Geometry check sheet. Reference: the model listing, model coordinates, mm. A direction names the side the tool comes from. Coordinates: 2 decimals unless noted, no trailing zeros. Write each loop counter-clockwise with the first axis right and the second up, starting at its lowest first coordinate (ties: lowest second). Pieces come first, ordered by that corner, then holes.
Autodesk Inventor part; units mm, degrees
ref_plane "Start Plane" through (0, 0, 0) normal (0, 0, 1) x (1, 0, 0)
ref_plane "End Plane" through (0, 0, 494.9747) normal (0, 0, 1) x (1, 0, 0)
ref_plane "Work Plane4" through (12.7, 0, 494.9747) normal (0, 0.3827, 0.9239) x (1, 0, 0)
ref_plane "Start Plane" through (0, 0, 0) normal (0, 0, 1) x (1, 0, 0)
ref_plane "End Plane" through (0, 0, 494.9747) normal (0, 0, 1) x (1, 0, 0)
sketch "Sketch" plane through (0, 0, 0) normal (0, 0, 1) x (1, 0, 0)
  line L0 (25.4, 0) -> (0, 0)
  line L1 (0, 0) -> (0, 25.4)
  line L2 (0, 25.4) -> (1.651, 25.4)
  line L3 (3.175, 23.876) -> (3.175, 6.477)
  line L4 (6.477, 3.175) -> (23.876, 3.175)
  line L5 (25.4, 1.651) -> (25.4, 0)
  line L6 (0, -11.0414) -> (0, 31.5385) construction
  line L7 (-11.0414, 0) -> (31.5385, 0) construction
  arc A0 (3.175, 6.477) -> (6.477, 3.175) centre (6.477, 6.477) ccw
  arc A1 (3.175, 23.876) -> (1.651, 25.4) centre (1.651, 23.876) ccw
  arc A2 (25.4, 1.651) -> (23.876, 3.175) centre (23.876, 1.651) ccw
  line L8 (0, 40.0545) -> (0, -19.5574) construction
  line L9 (-19.5574, 0) -> (40.0545, 0) construction
  point P0 (3.175, 25.4)
  point P1 (3.175, 3.175)
  point P2 (25.4, 3.175)
  dimension "d0" = 25.4
  dimension "d1" = 25.4
  dimension "d2" = 3.175
  dimension "d3" = 3.175
  dimension "d10" = 0
  dimension "d11" = 0
  dimension "d14" = 3.302
  dimension "d15" = 1.524
extrude "Body" add sketch "Sketch" along normal up to surface (494.9747 mm away) from surface at 0
sketch "Sketch3" plane through (0, 0, 0) normal (0, 0, 1) x (1, 0, 0)
  line L0 (0, 0) -> (10, 0)
ref_plane "Work Plane3" through (0, 0, 0) normal (0, -1, 0) x (1, 0, 0)
ref_plane "Work Plane4" through (12.7, 0, 494.9747) normal (0, 0.3827, 0.9239) x (1, 0, 0)
split "Split1" plane through (12.7, 0, 494.9747) removes the side toward (0, 0.3827, 0.9239)
ref_plane "Work Plane5" through (0, 0, 0) normal (0, 0.7071, -0.7071) x (1, 0, 0)
split "Split2" plane through (0, 0, 0) removes the side toward (0, 0.7071, -0.7071)
sketch "Sketch4" plane through (0, 0, 0) normal (0, -1, 0) x (1, 0, 0)
  line L0 (-2, 0) -> (12, 0)
  line L1 (-2, 494.9747) -> (12, 494.9747)
  dimension "d17" = 494.9747
equation "\"d0\" = G_H"
equation "\"d1\" = G_H"
equation "\"d2\" = G_T"
equation "\"d3\" = G_T"
equation "\"d14\" = G_IR"
equation "\"d15\" = G_ER"
equation "\"d4\" = G_L"
equation "\"G_H\" = 25.4"
equation "\"G_T\" = 3.175"
equation "\"G_ER\" = 1.524"
equation "\"G_IR\" = 3.302"
equation "\"G_L\" = d17"
equation "\"ex\" = 0"
equation "\"G_OFFSET_START\" = 0"
equation "\"G_OFFSET_END\" = 0"
equation "\"d13\" = G_OFFSET_END + B_L"
equation "\"B_L\" = 494.97475"
properties part number "AISC - L 1 x 1 x 1/8 - 19.487" material "Steel, Mild"
1. Sectioned sample at C-C, the plane y = 17.5. Record the boundary of the cut face in (x, z) (3 decimals), and give its area (3 significant figures).
Computed values:
outline: (0, 17.5) - (3.175, 17.5) - (3.175, 487.726) - (0, 487.726) - close
area: 1,490 mm2
2. Sectioned sample at A-A, the plane z = 306. Record the boundary of the cut face in (x, y) (3 decimals), and give its area (3 significant figures).
Computed values:
outline: (0, 0) - (25.4, 0) - (25.4, 1.651) arc R1.524 ccw to (23.876, 3.175) - (6.477, 3.175) arc R3.302 cw to (3.175, 6.477) - (3.175, 23.876) arc R1.524 ccw to (1.651, 25.4) - (0, 25.4) - close
area: 153 mm2
3. Thickness scan on line 1 along X through (y, z) = (10.75, 29.5) (3 decimals); line 2 along Z through (x, y) = (1, 22). Record the ranges inside material, lowest first.
Computed values:
line 1: x = 0 to 3.175
line 2: z = 22 to 485.86
4. Access from +Z, -Z, +X, -X, +Y, -Y to the whole of each face (thin tool, end or side, straight path). Record for faces 1 (the flat face through (3.175, 15, 246)), 2 (the flat face through (2, 8, 8)).
Computed values:
face 1: +Z, -Z, +X, +Y
face 2: -Z, +X, -X, +Y
5. Sectioned sample at B-B, the plane x = 19.75. Record the boundary of the cut face in (y, z) (3 decimals), and give its area (3 significant figures).
Computed values:
outline: (0, 0) - (3.175, 3.175) - (3.175, 493.66) - (0, 494.975) - close
area: 1,560 mm2
6. Gauge pin test, flat ends, axial feed: pin 1 Ø6 at (x, y) = (2.5, 22.5) entering from +Z; pin 2 Ø1 at (x, z) = (14, 122.5) entering from +Y (3 decimals); pin 3 Ø1.5 at (x, y) = (19, 3) entering from -Z; pin 4 Ø5 at (y, z) = (3, 414) entering from +X. Record the tip position at first contact, or that the pin passes through.
Computed values:
pin 1: stops at z = 486.9
pin 2: stops at y = 3.175
pin 3: stops at z = 2.25
pin 4: stops at x = 25.4
